CAD build for the part. Positions are in the model's coordinates, mm. Give positions to 0.01 mm unless a question says otherwise; leave off trailing zeros. Loops run counter-clockwise (first coordinate to the right, second up) from the corner with the lowest first, then second, coordinate; pieces in that order, holes last. Notation, with made-up numbers: (71.5, 53.5) -> (102.5, 53.5) arc R22 ccw to (102.5, 62.5) -> close; hole circle Ø11 at (-38, 52.25). An arc over 180 degrees is marked (long way). Use one line per item in the form item = value.
```python
from build123d import *

# Parameters (mm, degrees)
F1_DEPTH = 18
F2_DEPTH = 9


# Not quite as in the source:
# - ends of sketch curves that miss each other by under 0.0002 mm in the source are joined


with BuildPart() as f1:
    # F0 (on Top) → F1 (new body)
    with BuildSketch(Plane.XY):
        with BuildLine():
            Line((-1127.3931139915, 97.8692322969), (-1127.3931139915, -62.1307669387))
            Line((-1127.3931139915, -62.1307669387), (-930.8931139915, -62.1307669387))
            ThreePointArc((-930.8931139915, -62.1307669387), (-924.9182402574, -59.6558932046), (-927.3931139915, -65.6307669387))
            Line((-927.3931139915, -65.6307669387), (-927.3931139915, -80.1307669387))
            Line((-927.3931139915, -80.1307669387), (-777.3931378334, -80.1307669387))
            Line((-777.3931378334, -80.1307669387), (-777.3931378334, -65.6307669387))
            ThreePointArc((-777.3931378334, -65.6307669387), (-779.8680115675, -59.6558932046), (-773.8931378334, -62.1307669387))
            Line((-773.8931378334, -62.1307669387), (-630.8931139915, -62.1307669387))
            ThreePointArc((-630.8931139915, -62.1307669387), (-624.9182402574, -59.6558932046), (-627.3931139915, -65.6307669387))
            Line((-627.3931139915, -65.6307669387), (-627.3931139915, -80.1307669387))
            Line((-627.3931139915, -80.1307669387), (-477.3931378334, -80.1307669387))
            Line((-477.3931378334, -80.1307669387), (-477.3931378334, -65.6307669387))
            ThreePointArc((-477.3931378334, -65.6307669387), (-479.8680115675, -59.6558932046), (-473.8931378334, -62.1307669387))
            Line((-473.8931378334, -62.1307669387), (-330.8931139915, -62.1307669387))
            ThreePointArc((-330.8931139915, -62.1307669387), (-324.9182402574, -59.6558932046), (-327.3931139915, -65.6307669387))
            Line((-327.3931139915, -65.6307669387), (-327.3931139915, -80.1307669387))
            Line((-327.3931139915, -80.1307669387), (-177.3931378334, -80.1307669387))
            Line((-177.3931378334, -80.1307669387), (-177.3931378334, -65.6307669387))
            ThreePointArc((-177.3931378334, -65.6307669387), (-179.8680115675, -59.6558932046), (-173.8931378334, -62.1307669387))
            Line((-173.8931378334, -62.1307669387), (-27.3931378334, -62.1307669387))
            Line((-27.3931378334, -62.1307669387), (119.1069098503, -62.1307669387))
            ThreePointArc((119.1069098503, -62.1307669387), (125.0817835845, -59.6558932046), (122.6069098503, -65.6307669387))
            Line((122.6069098503, -65.6307669387), (122.6069098503, -80.1307669387))
            Line((122.6069098503, -80.1307669387), (272.6068860085, -80.1307669387))
            Line((272.6068860085, -80.1307669387), (272.6068860085, -65.6307669387))
            ThreePointArc((272.6068860085, -65.6307669387), (270.1320122743, -59.6558932046), (276.1068860085, -62.1307669387))
            Line((276.1068860085, -62.1307669387), (419.1069098503, -62.1307669387))
            ThreePointArc((419.1069098503, -62.1307669387), (425.0817835845, -59.6558932046), (422.6069098503, -65.6307669387))
            Line((422.6069098503, -65.6307669387), (422.6069098503, -80.1307669387))
            Line((422.6069098503, -80.1307669387), (572.6068860085, -80.1307669387))
            Line((572.6068860085, -80.1307669387), (572.6068860085, -65.6307669387))
            ThreePointArc((572.6068860085, -65.6307669387), (570.1320122743, -59.6558932046), (576.1068860085, -62.1307669387))
            Line((576.1068860085, -62.1307669387), (719.1069098503, -62.1307669387))
            ThreePointArc((719.1069098503, -62.1307669387), (725.0817835845, -59.6558932046), (722.6069098503, -65.6307669387))
            Line((722.6069098503, -65.6307669387), (722.6069098503, -80.1307669387))
            Line((722.6069098503, -80.1307669387), (872.6068860085, -80.1307669387))
            Line((872.6068860085, -80.1307669387), (872.6068860085, -65.6307669387))
            ThreePointArc((872.6068860085, -65.6307669387), (870.1320122743, -59.6558932046), (876.1068860085, -62.1307669387))
            Line((876.1068860085, -62.1307669387), (1072.6068860085, -62.1307669387))
            Line((1072.6068860085, -62.1307669387), (1072.6068860085, 97.8692322969))
            Line((1072.6068860085, 97.8692322969), (1072.6068860085, 257.8692315326))
            Line((1072.6068860085, 257.8692315326), (876.1068860085, 257.8692315326))
            ThreePointArc((876.1068860085, 257.8692315326), (870.1320122743, 255.3943577985), (872.6068860085, 261.3692315326))
            Line((872.6068860085, 261.3692315326), (872.6068860085, 275.8692315326))
            Line((872.6068860085, 275.8692315326), (722.6069098503, 275.8692315326))
            Line((722.6069098503, 275.8692315326), (722.6069098503, 261.3692315326))
            ThreePointArc((722.6069098503, 261.3692315326), (725.0817835845, 255.3943577985), (719.1069098503, 257.8692315326))
            Line((719.1069098503, 257.8692315326), (576.1068860085, 257.8692315326))
            ThreePointArc((576.1068860085, 257.8692315326), (570.1320122743, 255.3943577985), (572.6068860085, 261.3692315326))
            Line((572.6068860085, 261.3692315326), (572.6068860085, 275.8692315326))
            Line((572.6068860085, 275.8692315326), (422.6069098503, 275.8692315326))
            Line((422.6069098503, 275.8692315326), (422.6069098503, 261.3692315326))
            ThreePointArc((422.6069098503, 261.3692315326), (425.0817835845, 255.3943577985), (419.1069098503, 257.8692315326))
            Line((419.1069098503, 257.8692315326), (276.1068860085, 257.8692315326))
            ThreePointArc((276.1068860085, 257.8692315326), (270.1320122743, 255.3943577985), (272.6068860085, 261.3692315326))
            Line((272.6068860085, 261.3692315326), (272.6068860085, 275.8692315326))
            Line((272.6068860085, 275.8692315326), (122.6069098503, 275.8692315326))
            Line((122.6069098503, 275.8692315326), (122.6069098503, 261.3692315326))
            ThreePointArc((122.6069098503, 261.3692315326), (125.0817835845, 255.3943577985), (119.1069098503, 257.8692315326))
            Line((119.1069098503, 257.8692315326), (-27.3930901497, 257.8692315326))
            Line((-27.3930901497, 257.8692315326), (-173.8931378334, 257.8692315326))
            ThreePointArc((-173.8931378334, 257.8692315326), (-179.8680115675, 255.3943577985), (-177.3931378334, 261.3692315326))
            Line((-177.3931378334, 261.3692315326), (-177.3931378334, 275.8692315326))
            Line((-177.3931378334, 275.8692315326), (-327.3931139915, 275.8692315326))
            Line((-327.3931139915, 275.8692315326), (-327.3931139915, 261.3692315326))
            ThreePointArc((-327.3931139915, 261.3692315326), (-324.9182402574, 255.3943577985), (-330.8931139915, 257.8692315326))
            Line((-330.8931139915, 257.8692315326), (-473.8931378334, 257.8692315326))
            ThreePointArc((-473.8931378334, 257.8692315326), (-479.8680115675, 255.3943577985), (-477.3931378334, 261.3692315326))
            Line((-477.3931378334, 261.3692315326), (-477.3931378334, 275.8692315326))
            Line((-477.3931378334, 275.8692315326), (-627.3931139915, 275.8692315326))
            Line((-627.3931139915, 275.8692315326), (-627.3931139915, 261.3692315326))
            ThreePointArc((-627.3931139915, 261.3692315326), (-624.9182402574, 255.3943577985), (-630.8931139915, 257.8692315326))
            Line((-630.8931139915, 257.8692315326), (-773.8931378334, 257.8692315326))
            ThreePointArc((-773.8931378334, 257.8692315326), (-779.8680115675, 255.3943577985), (-777.3931378334, 261.3692315326))
            Line((-777.3931378334, 261.3692315326), (-777.3931378334, 275.8692315326))
            Line((-777.3931378334, 275.8692315326), (-927.3931139915, 275.8692315326))
            Line((-927.3931139915, 275.8692315326), (-927.3931139915, 261.3692315326))
            ThreePointArc((-927.3931139915, 261.3692315326), (-924.9182402574, 255.3943577985), (-930.8931139915, 257.8692315326))
            Line((-930.8931139915, 257.8692315326), (-1127.3931139915, 257.8692315326))
            Line((-1127.3931139915, 257.8692315326), (-1127.3931139915, 97.8692322969))
        make_face()
        with BuildLine():
            Line((-22.8931139915, 190.8692322969), (-22.8931139915, 97.8692322969))
            Line((-22.8931139915, 97.8692322969), (-22.8931139915, 4.8692322969))
            ThreePointArc((-22.8931139915, 4.8692322969), (-19.3931139915, 1.3692322969), (-22.8931139915, -2.1307677031))
            Line((-22.8931139915, -2.1307677031), (-27.3931139915, -2.1307677031))
            Line((-27.3931139915, -2.1307677031), (-31.8931139915, -2.1307677031))
            ThreePointArc((-31.8931139915, -2.1307677031), (-35.3931139915, 1.3692322969), (-31.8931139915, 4.8692322969))
            Line((-31.8931139915, 4.8692322969), (-31.8931139915, 97.8692322969))
            Line((-31.8931139915, 97.8692322969), (-31.8931139915, 190.8692322969))
            ThreePointArc((-31.8931139915, 190.8692322969), (-35.3931139915, 194.3692322969), (-31.8931139915, 197.8692322969))
            Line((-31.8931139915, 197.8692322969), (-27.3931139915, 197.8692322969))
            Line((-27.3931139915, 197.8692322969), (-22.8931139915, 197.8692322969))
            ThreePointArc((-22.8931139915, 197.8692322969), (-19.3931139915, 194.3692322969), (-22.8931139915, 190.8692322969))
        make_face(mode=Mode.SUBTRACT)
    extrude(amount=F1_DEPTH)

    # F0 (on Top) → F2 (join)
    with BuildSketch(Plane.XY):
        with BuildLine():
            Line((-22.8931139915, 4.8692322969), (-22.8931139915, 97.8692322969))
            Line((-22.8931139915, 97.8692322969), (-22.8931139915, 190.8692322969))
            ThreePointArc((-22.8931139915, 190.8692322969), (-19.3931139915, 194.3692322969), (-22.8931139915, 197.8692322969))
            Line((-22.8931139915, 197.8692322969), (-27.3931139915, 197.8692322969))
            Line((-27.3931139915, 197.8692322969), (-31.8931139915, 197.8692322969))
            ThreePointArc((-31.8931139915, 197.8692322969), (-35.3931139915, 194.3692322969), (-31.8931139915, 190.8692322969))
            Line((-31.8931139915, 190.8692322969), (-31.8931139915, 97.8692322969))
            Line((-31.8931139915, 97.8692322969), (-31.8931139915, 4.8692322969))
            ThreePointArc((-31.8931139915, 4.8692322969), (-35.3931139915, 1.3692322969), (-31.8931139915, -2.1307677031))
            Line((-31.8931139915, -2.1307677031), (-27.3931139915, -2.1307677031))
            Line((-27.3931139915, -2.1307677031), (-22.8931139915, -2.1307677031))
            ThreePointArc((-22.8931139915, -2.1307677031), (-19.3931139915, 1.3692322969), (-22.8931139915, 4.8692322969))
        make_face()
    extrude(amount=F2_DEPTH)


solid = f1.part
```
1. Cut at A-A, the plane x = 614. Write the cut outline in (y, z), then the cut area to 3 significant figures.
Result sheet:
outline = (-62.13, 0) -> (257.87, 0) -> (257.87, 18) -> (-62.13, 18) -> close
area = 5,760 mm^2
2. Drill centre lines: line 1 (X direction, y = 258, z = 1.75); line 2 (X direction, y = 77.5, z = 16.5); line 3 (Y direction, x = 118.5, z = 6.5). Where is each one in solid material? Low to high.
Result sheet:
line_1 = -923.9 to -780.89, -623.9 to -480.89, -323.9 to -180.89, 126.1 to 269.11, 426.1 to 569.11, 726.1 to 869.11
line_2 = -1127.39 to -31.89, -22.89 to 1072.61
line_3 = -62.13 to 257.87
3. Drop flat-ended pins along their axis: P1, Ø4, axis at x = 272.61, y = -62.13, coming from the -Z side; P2, Ø1, axis at x = -357, z = 11, coming from the -Y side; P3, Ø5.5, axis at x = 618, z = 4.5, coming from the +Y side; P4, Ø4.5, axis at y = -70.5, z = 11.5, coming from the +X side. Give the stop position or say it passes through.
Result sheet:
P1 = through
P2 = -62.13
P3 = 257.87
P4 = 872.61
